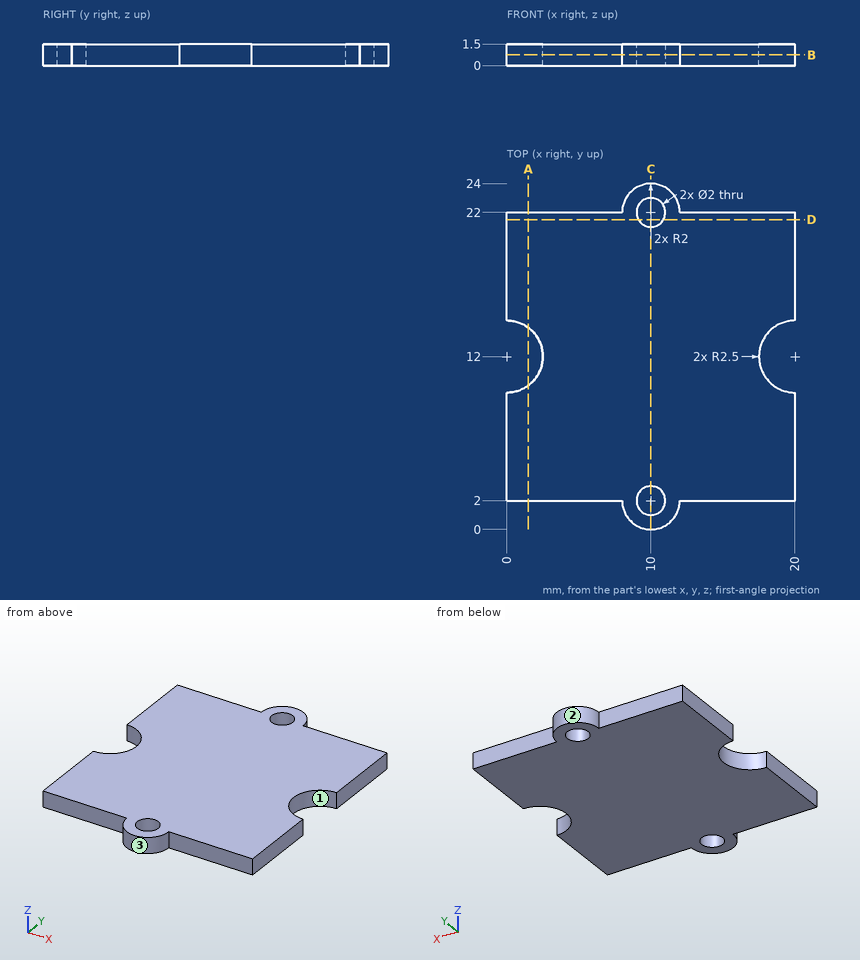
Geometry check sheet. Reference: drawing and pictorial views, mm from the part's lowest x, y, z. Give positions to 0.01 mm unless a question says otherwise; leave off trailing zeros. Order: outer loops, then holes, each group sorted by start corner. A loop starts at its lowest first (then second) coordinate and runs counter-clockwise, first axis right, second up. Notation, with made-up numbers: M 39.5,-27.75 L 44.5,-27.75 A24 cw 44.5,-5.75 Z; hole C -5,52 d10. An arc over 180 degrees is marked long. Answer as CSV lines item,"result". Start each with the question number.
Item 1: Cross-section at D-D on y = 21.5. Enter the section's corners in (x, z), plus the area to 3 significant figures.
Item 2: Mould release check, pull along Y, two halves, no side actions. Record for the marked faces 1, 2 and 3: +Y half, -Y half, draft (parallel to the pull), parting line (faces both ways), or undercut.
Item 3: Thickness scan on line 1 (Y direction, x = 10, z = 1.15); line 2 (Y direction, x = 15.5, z = 0.85); line 3 (Y direction, x = 1.25, z = 1). Record the ranges inside material, lowest first. Write a range as [from, to].
Item 4: Cross-section at A-A on x = 1.5. Enter the section's corners in (y, z).
Item 5: Cross-section at C-C on x = 10. Enter the section's corners in (y, z), plus the area to 3 significant figures.
Item 6: Cross-section at B-B on z = 0.75. Enter the section's corners in (x, y), plus the area to 3 significant figures.
Item 7: Gauge pin test, flat end, axial feed: P1, Ø0.8, axis at x = 15.5, z = 0.5, coming from the -Y side. Record the tip position at first contact, or that the pin passes through.
Established:
1,outline,"M 0,0 L 9.13,0 L 9.13,1.5 L 0,1.5 Z; M 10.87,0 L 20,0 L 20,1.5 L 10.87,1.5 Z"
1,area,"27.4 mm^2"
2,face 1,"undercut"
2,face 2,"+Y half"
2,face 3,"-Y half"
3,line 1,"y = [0, 1], [3, 21], [23, 24]"
3,line 2,"y = [2, 22]"
3,line 3,"y = [2, 9.83], [14.17, 22]"
4,outline,"M 2,0 L 10,0 L 10,1.5 L 2,1.5 Z; M 14,0 L 22,0 L 22,1.5 L 14,1.5 Z"
5,outline,"M 0,0 L 1,0 L 1,1.5 L 0,1.5 Z; M 3,0 L 21,0 L 21,1.5 L 3,1.5 Z; M 23,0 L 24,0 L 24,1.5 L 23,1.5 Z"
5,area,"30.0 mm^2"
6,outline,"M 0,2 L 8,2 A2 ccw 12,2 L 20,2 L 20,9.5 A2.5 cw 20,14.5 L 20,22 L 12,22 A2 ccw 8,22 L 0,22 L 0,14.5 A2.5 cw 0,9.5 Z; hole C 10,2 d2; hole C 10,22 d2"
6,area,"387 mm^2"
7,P1,"stops at y = 2"
